Could you check a few things on this model? Use its own coordinates, in mm. A direction names the side the tool comes from. Give positions to 0.01 mm unless a question says otherwise; leave off trailing zeros. Order: outer loops, then holes, each group sorted by start corner. A loop starts at its lowest first (then second) coordinate and runs counter-clockwise, first axis right, second up. Notation, with made-up numbers: (-18.5, -24.5) - (39.5, -24.5) arc R24 ccw to (39.5, -9.5) - close; hole circle Ø1 at (66, 10). An arc over 180 degrees is marked (long way). Put each result on its own line as item: value.
Solid Edge part; units mm, degrees
sketch "Sketch1" plane through (0, 0, 0) normal (0, 0, 1) x (1, 0, 0)
  line L0 (7.5, -5.2) -> (7.5, 5.2)
  line L1 (7.5, 5.2) -> (-7.5, 5.2)
  line L2 (-7.5, 5.2) -> (-7.5, -5.2)
  line L3 (-7.5, -5.2) -> (7.5, -5.2)
extrude "Protrusion1" add sketch "Sketch1" along normal blind 1.5
sketch "Sketch2" plane through (0, 0, 0) normal (0, 0, 1) x (1, 0, 0)
  line L0 (6.5, 4.2) -> (-6.5, 4.2)
  line L1 (-6.5, 4.2) -> (-6.5, -4.2)
  line L2 (-6.5, -4.2) -> (6.5, -4.2)
  line L3 (6.5, -4.2) -> (6.5, 4.2)
extrude "ExtrudedProtrusion_2" add sketch "Sketch2" against normal blind 9
sketch "Sketch3" plane through (0, 0, -9) normal (0, 0, -1) x (1, 0, 0)
  line L0 (-0.25, 2.75) -> (-0.25, -2.75)
  line L1 (-0.25, -2.75) -> (0.25, -2.75)
  line L2 (0.25, -2.75) -> (0.25, 2.75)
  line L3 (0.25, 2.75) -> (-0.25, 2.75)
  line L4 (5.25, -2.75) -> (5.25, 2.75)
  line L5 (5.25, 2.75) -> (4.75, 2.75)
  line L6 (4.75, 2.75) -> (4.75, -2.75)
  line L7 (4.75, -2.75) -> (5.25, -2.75)
extrude "ExtrudedProtrusion_3" add sketch "Sketch3" along normal blind 7
sketch "Sketch4" plane through (0, 0, 0) normal (0, -1, 0) x (1, 0, 0)
  line L0 (-4.8786, 3.5) -> (4.8786, 1.5)
  line L1 (4.8786, 1.5) -> (-4.8786, 1.5)
  line L2 (-4.8786, 1.5) -> (-4.8786, 3.5)
extrude "ExtrudedProtrusion_4" add sketch "Sketch4" along normal mid plane 8
properties material "Graphite"
1) Suppose I cut it at A-A, the plane z = -10. List the corners of the cut face in (x, y) for me, and give its area (3 significant figures).
Filled in:
outline: (-0.25, -2.75) - (0.25, -2.75) - (0.25, 2.75) - (-0.25, 2.75) - close; (4.75, -2.75) - (5.25, -2.75) - (5.25, 2.75) - (4.75, 2.75) - close
area: 5.50 mm^2
2) Suppose I cut it at B-B, the plane y = 1.75. List the corners of the cut face in (x, z) for me.
Filled in:
outline: (-7.5, 0) - (-6.5, 0) - (-6.5, -9) - (-0.25, -9) - (-0.25, -16) - (0.25, -16) - (0.25, -9) - (4.75, -9) - (4.75, -16) - (5.25, -16) - (5.25, -9) - (6.5, -9) - (6.5, 0) - (7.5, 0) - (7.5, 1.5) - (4.88, 1.5) - (-4.88, 3.5) - (-4.88, 1.5) - (-7.5, 1.5) - close
3) Which directions (+Z, -Z, +X, -X, +Y, -Y) give clear straight access to the entire face, cutting with the end or side of a thin tool? Please do faces 5 (the flat face through (4.75, 0, -12)), 6 (the flat face through (-2, 4, 2)), 7 (the flat face through (0, 4.2, -4)).
Filled in:
face 5: -Z, +Y, -Y
face 6: +Z, +X, -X, +Y
face 7: -Z, +X, -X, +Y
4) We'd pull the mould along X, two halves only. Please class faces 1 (the flat face through (0, -5, 0)), 2 (the flat face through (5.25, 0, -12)), 3 (the flat face through (0.25, 0, -12)), 4 (the flat face through (-0.25, 0, -12)): pulls with the +X half, pulls with the -X half, needs draft (parallel to the pull), parting line crosses it, or undercut.
Filled in:
face 1: needs draft
face 2: pulls with the +X half
face 3: undercut
face 4: pulls with the -X half
5) I'm going to push flat-ended pins straight in: pin 1 (1 mm diameter, centred on y = 1, z = -6.5, fed in from +X); pin 2 (2.5 mm diameter, centred on x = 3, z = -4.5, fed in from -Y); pin 3 (0.6 mm diameter, centred on x = 0, z = -14, fed in from -Y). Where does each tip first touch, or does it pass through?
Filled in:
pin 1: stops at x = 6.5
pin 2: stops at y = -4.2
pin 3: stops at y = -2.75
6) If I drill on line 1 (X direction, y = 0.25, z = -12); line 2 (Y direction, x = 4.75, z = -7.5); line 3 (Z direction, x = 4, y = -4.5), over which ranges is the centre line in solid material (lowest first)? Write a range as [from, to].
Filled in:
line 1: x = [-0.25, 0.25], [4.75, 5.25]
line 2: y = [-4.2, 4.2]
line 3: z = [0, 1.5]
7) Suppose I cut it at D-D, the plane z = -3.25. List the corners of the cut face in (x, y) for me, and give its area (3 significant figures).
Filled in:
outline: (-6.5, -4.2) - (6.5, -4.2) - (6.5, 4.2) - (-6.5, 4.2) - close
area: 109 mm^2
8) Suppose I cut it at C-C, the plane x = -3.75. List the corners of the cut face in (y, z) for me.
Filled in:
outline: (-5.2, 0) - (-4.2, 0) - (-4.2, -9) - (4.2, -9) - (4.2, 0) - (5.2, 0) - (5.2, 1.5) - (4, 1.5) - (4, 3.27) - (-4, 3.27) - (-4, 1.5) - (-5.2, 1.5) - close
